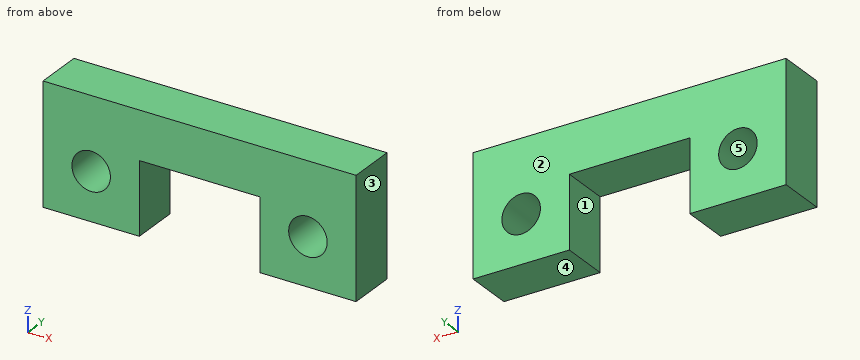
```python
from build123d import *

# Parameters (mm, degrees)
BOSS_EXTRUDE1_DEPTH = 5
SKETCH2_R           = 4
CUT_EXTRUDE1_DEPTH  = 43.20485754


with BuildPart() as part:
    # Sketch1 → Boss-Extrude1 (new, symmetric)
    with BuildSketch(Plane(origin=(0, 0, 0), x_dir=(1, 0, 0), z_dir=(0, 1, 0))):
        Polygon((32.5, 0), (-32.5, 0), (-32.5, 25), (-12.5, 25), (-12.5, 10), (12.5, 10), (12.5, 25), (32.5, 25), align=None)
    extrude(amount=BOSS_EXTRUDE1_DEPTH, both=True)

    # Sketch2 → Cut-Extrude1 (cut, symmetric)
    with BuildSketch(Plane(origin=(0, 5, 0), x_dir=(1, 0, 0), z_dir=(0, 1, 0))):
        with Locations(Location((-22.5, 15, 0), (0, 0, 270))):
            Circle(SKETCH2_R)
    cut_extrude1 = extrude(amount=CUT_EXTRUDE1_DEPTH, both=True, mode=Mode.SUBTRACT)

    # Mirror1: Cut-Extrude1 across plane
    add(cut_extrude1.mirror(Plane(origin=(0, 0, 0), x_dir=(0, 0, 1), z_dir=(1, 0, 0))), mode=Mode.SUBTRACT)


solid = part.part
```
Model file for the job. Use its own axes, mm. Face numbers are marked on the shaded views. A direction names the side the tool comes from. Coordinates: 2 decimals unless noted, no trailing zeros. Loops run counter-clockwise (first coordinate to the right, second up) from the corner with the lowest first, then second, coordinate; pieces in that order, holes last. Notation, with made-up numbers: (18.25, 52.5) -> (30.25, 52.5) arc R25 ccw to (30.25, 75.5) -> close; hole circle Ø9 at (51.5, -16). An arc over 180 degrees is marked (long way). Answer as a JSON object with one key per item and string values.
Q1. Probe probe 1 along X at (y, z) = (1.25, -15); probe 2 along X at (y, z) = (-4, -11.5); probe 3 along Z at (x, y) = (5.5, -1.75). List the from-to ranges inside material, lowest first.
Report:
{"probe 1": "x = -32.5 to -26.5, -18.5 to -12.5, 12.5 to 18.5, 26.5 to 32.5", "probe 2": "x = -32.5 to -24.44, -20.56 to -12.5, 12.5 to 20.56, 24.44 to 32.5", "probe 3": "z = -10 to 0"}
Q2. Cut at A-A (y = -1). List the corners of the cut face in (x, z).
Report:
{"outline": "(-32.5, -25) -> (-12.5, -25) -> (-12.5, -10) -> (12.5, -10) -> (12.5, -25) -> (32.5, -25) -> (32.5, 0) -> (-32.5, 0) -> close; hole circle Ø8 at (-22.5, -15); hole circle Ø8 at (22.5, -15)"}
Q3. Cut at B-B (z = -22). List the corners of the cut face in (x, y), and give its area (3 significant figures).
Report:
{"outline": "(-32.5, -5) -> (-12.5, -5) -> (-12.5, 5) -> (-32.5, 5) -> close; (12.5, -5) -> (32.5, -5) -> (32.5, 5) -> (12.5, 5) -> close", "area": "400 mm2"}
Q4. 3-axis set-ups, long thin cutter, end or side, ignore diameter. For the marked faces 1 and 2: which of +Z, -Z, +X, -X, +Y, -Y reach the whole face in a straight line?
Report:
{"face 1": "-Z, +Y, -Y", "face 2": "+Z, -Z, +X, -X, +Y"}
Q5. Flat gauge pins, fed straight in: P1, Ø4, axis at x = -7, z = -13.5, coming from the +Y side; P2, Ø5, axis at x = 6.5, y = 1, coming from the -Z side. Where does each tip first touch, or does it go through?
Report:
{"P1": "passes through", "P2": "stops at z = -10"}
Q6. Cut at C-C (x = -22.5). List the corners of the cut face in (y, z), and give its area (3 significant figures).
Report:
{"outline": "(-5, -25) -> (5, -25) -> (5, -19) -> (-5, -19) -> close; (-5, -11) -> (5, -11) -> (5, 0) -> (-5, 0) -> close", "area": "170 mm2"}
Q7. Pull direction Z, two halves, no side cores. Call the marked faces 3, 4 and 5: released by +Z, released by -Z, zero draft, split by the parting line, or undercut.
Report:
{"face 3": "zero draft", "face 4": "released by -Z", "face 5": "undercut"}
Q8. Cut at D-D (x = -9). List the corners of the cut face in (y, z), and give its area (3 significant figures).
Report:
{"outline": "(-5, -10) -> (5, -10) -> (5, 0) -> (-5, 0) -> close", "area": "100 mm2"}
